from build123d import *

# Parameters (mm, degrees)
BOSS_EXTRUDE1_DEPTH = 4.7625


with BuildPart() as part:
    # Sketch1 → Boss-Extrude1 (new body)
    with BuildSketch(Plane.XY):
        with BuildLine():
            Line((-7.45, 3), (0, 3))
            Line((0, 3), (0, 0))
            Line((0, 0), (-7.45, 0))
            Line((-7.45, 0), (-7.45, -1))
            Line((-7.45, -1), (-5.95, -1))
            ThreePointArc((-5.95, -1), (-6.389339828, -2.060660172), (-7.45, -2.5))
            ThreePointArc((-7.45, -2.5), (-10.2, 0.25), (-7.45, 3))
        make_face()
    boss_extrude1 = extrude(amount=BOSS_EXTRUDE1_DEPTH)

    # Mirror1: Boss-Extrude1 across plane
    add(boss_extrude1.mirror(Plane(origin=(0, 0, 4.7625), x_dir=(0, 0, 1), z_dir=(-1, 0, 0))))


solid = part.part
Geometry: final body of the model. Coordinates: model frame, mm. A direction names the side the tool comes from. Give positions to 0.01 mm unless a question says otherwise; leave off trailing zeros. Write each loop counter-clockwise with the first axis right and the second up, starting at its lowest first coordinate (ties: lowest second). Pieces come first, ordered by that corner, then holes. Notation, with made-up numbers: (-11, -5.5) -> (33, -5.5) arc R9 cw to (33, 9.5) -> close; hole circle Ø2 at (73.5, 50). An arc over 180 degrees is marked (long way). Answer as a JSON object with one key per item and string values.
1. Ray query, probe 1 along Y at (x, z) = (-2.5, 3.4); probe 2 along X at (y, z) = (-1.95, 2.5); probe 3 along X at (y, z) = (-0.4, 2.75). Return the intervals inside material, ascending. Write a range as from..to.
Ans:
{"probe 1": "y = 0..3", "probe 2": "x = -9.1..-6.29, 6.29..9.1", "probe 3": "x = -10.12..-7.45, 7.45..10.12"}
2. Cut plane C-C on x = -4.25. Output: boundary loops of the cut face in (y, z), and give its area (3 significant figures).
Ans:
{"outline": "(0, 0) -> (3, 0) -> (3, 4.76) -> (0, 4.76) -> close", "area": "14.3 mm^2"}
3. Cut plane A-A on y = -2.1. Output: boundary loops of the cut face in (x, z).
Ans:
{"outline": "(-8.88, 0) -> (-6.43, 0) -> (-6.43, 4.76) -> (-8.88, 4.76) -> close; (6.43, 0) -> (8.88, 0) -> (8.88, 4.76) -> (6.43, 4.76) -> close"}
4. Mould query, pull axis Y, two halves, no side actions, for faces 1 (the cylindrical face through (-6.38, -2.05, 2.35)), 2 (the flat face through (0, 1, 0)), 3 (the flat face through (-7, -1, 2)). Classes: pulls with the +Y half, pulls with the -Y half, needs draft (parallel to the pull), parting line crosses it, or undercut.
Ans:
{"face 1": "pulls with the -Y half", "face 2": "needs draft", "face 3": "undercut"}
5. Contact query for flat-ended pins moving along their axis: pin 1 (0.8 mm diameter, centred on y = -0.5, z = 2, fed in from +X); pin 2 (0.8 mm diameter, centred on y = -0.5, z = 2, fed in from -X); pin 3 (1.5 mm diameter, centred on y = 2, z = 1.5, fed in from +X). Output: stop coordinate, or through.
Ans:
{"pin 1": "stops at x = 10.18", "pin 2": "stops at x = -10.18", "pin 3": "stops at x = 10.01"}
6. Cut plane D-D on y = 2.65. Output: boundary loops of the cut face in (x, z).
Ans:
{"outline": "(-8.79, 0) -> (8.79, 0) -> (8.79, 4.76) -> (-8.79, 4.76) -> close"}
7. Access query for faces 4 (the cylindrical face through (6.38, -2.05, 2.35)), 5 (the flat face through (0, 1, 4.762)), 6 (the flat face through (7.45, -0.5, 2.3)). Directions: +Z, -Z, +X, -X, +Y, -Y. A direction counts if a zero-diameter tool reaches every point of the face in a straight line with its end or side. Return the directions, or none.
Ans:
{"face 4": "+Z, -Z, -Y", "face 5": "+Z, +X, -X, +Y, -Y", "face 6": "+Z, -Z"}
8. Cut plane B-B on z = 2.55. Output: boundary loops of the cut face in (x, y).
Ans:
{"outline": "(-7.45, -2.5) arc R1.5 ccw to (-5.95, -1) -> (-7.45, -1) -> (-7.45, 0) -> (7.45, 0) -> (7.45, -1) -> (5.95, -1) arc R1.5 ccw to (7.45, -2.5) arc R2.75 ccw to (7.45, 3) -> (-7.45, 3) arc R2.75 ccw to start"}
